```python
from build123d import *

# Parameters (mm, degrees)
BOSS_EXTRUDE1_DEPTH = 3
SKETCH2_R           = 1
CUT_EXTRUDE1_DEPTH  = 3
CUT_EXTRUDE2_DEPTH  = 3
SKETCH4_R           = 1
CUT_EXTRUDE3_DEPTH  = 3


with BuildPart() as part:
    # Sketch1 → Boss-Extrude1 (new body)
    with BuildSketch(Plane(origin=(0, 0, 0), x_dir=(1, 0, 0), z_dir=(0, 1, 0))):
        with BuildLine():
            Line((0, 24), (100, 24))
            ThreePointArc((100, 24), (124, 0), (100, -24))
            Line((100, -24), (0, -24))
            ThreePointArc((0, -24), (-24, 0), (0, 24))
        make_face()
    extrude(amount=BOSS_EXTRUDE1_DEPTH)

    # Sketch2 → Cut-Extrude1 (cut)
    with BuildSketch(Plane(origin=(0, 3, 0), x_dir=(1, 0, 0), z_dir=(0, 1, 0))):
        with Locations(Location((0, 0, 0), (0, 0, 270))):
            Circle(SKETCH2_R)
    extrude(amount=-CUT_EXTRUDE1_DEPTH, mode=Mode.SUBTRACT)

    # Sketch3 → Cut-Extrude2 (cut)
    with BuildSketch(Plane(origin=(0, 3, 0), x_dir=(1, 0, 0), z_dir=(0, 1, 0))):
        with BuildLine():
            Line((105.344155686, 2.5), (105.904155686, 2.5))
            ThreePointArc((105.904155686, 2.5), (108.404155686, 0), (105.904155686, -2.5))
            Line((105.904155686, -2.5), (105.344155686, -2.5))
            ThreePointArc((105.344155686, -2.5), (94.1, 0), (105.344155686, 2.5))
        make_face()
    extrude(amount=-CUT_EXTRUDE2_DEPTH, mode=Mode.SUBTRACT)

    # Sketch4 → Cut-Extrude3 (cut)
    with BuildSketch(Plane(origin=(0, 3, 0), x_dir=(1, 0, 0), z_dir=(0, 1, 0))):
        with Locations(Location((91.8, 0, 0), (0, 0, 270))):
            Circle(SKETCH4_R)
    extrude(amount=-CUT_EXTRUDE3_DEPTH, mode=Mode.SUBTRACT)


solid = part.part
```
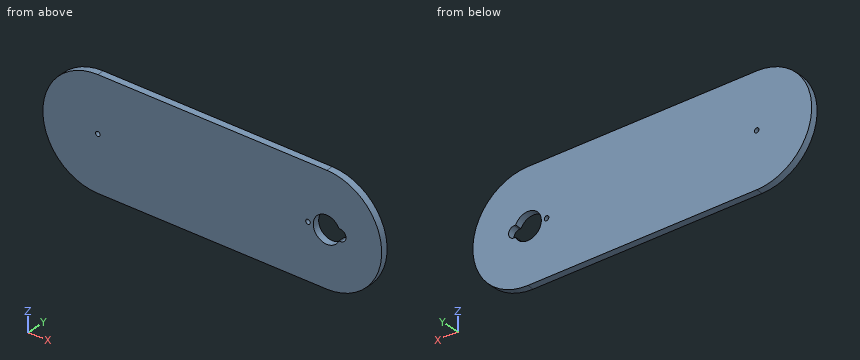
The model under review builds one solid part; all positions refer to its coordinate system, in mm. Round coordinates to 2 decimals unless told otherwise and drop trailing zeros. Loops run counter-clockwise (first coordinate to the right, second up) from the corner with the lowest first, then second, coordinate; pieces in that order, holes last. Notation, with made-up numbers: M 82.25,9.25 L 108.25,9.25 A13 cw 108.25,32.25 Z; hole C 47,73 d4. An arc over 180 degrees is marked long. Put each result on its own line as item: value.
Q1. Consider section C-C, the plane x = -5.5. Give the boundary of the cut face in (y, z).
Result set:
outline: M 0,-23.36 L 3,-23.36 L 3,23.36 L 0,23.36 Z
Q2. Consider section A-A, the plane y = 1.15. Give the boundary of the cut face in (x, z), then the cut area to 3 significant figures.
Result set:
outline: M 0,-24 L 100,-24 A24 ccw 100,24 L 0,24 A24 ccw Z; hole C 0,0 d2; hole C 91.8,0 d2; hole M 105.34,-2.5 L 105.9,-2.5 A2.5 ccw 105.9,2.5 L 105.34,2.5 A5.9 ccw long Z
area: 6,480 mm²
Q3. Consider section B-B, the plane z = -15. Give the boundary of the cut face in (x, y) (3 decimals), then the cut area to 3 significant figures.
Result set:
outline: M -18.735,0 L 118.735,0 L 118.735,3 L -18.735,3 Z
area: 412 mm²
Q4. To check wall thickness, follow L1, parallel to X at y = 0.75, z = 0; L2, parallel to Z at x = 91.8, y = 2.2; L3, parallel to Z at x = 100, y = 1.7. State the ranges of each line that lie inside material, in increasing order.
Result set:
L1: x = -24 to -1, 1 to 90.8, 92.8 to 94.1, 108.4 to 124
L2: z = -24 to -1, 1 to 24
L3: z = -24 to -5.9, 5.9 to 24
Q5. For pin 1 (1.6 mm diameter, centred on x = 91.8, z = 0, fed in from +Y), flat-tipped, find the tip position at first contact; note if it passes through.
Result set:
pin 1: passes through
